```python
from build123d import *

# Parameters (mm, degrees)
SKETCH1_R           = 45
BOSS_EXTRUDE1_DEPTH = 2
SKETCH2_R           = 45
SKETCH2_R_2         = 43
BOSS_EXTRUDE2_DEPTH = 60
BOSS_EXTRUDE3_DEPTH = 20


with BuildPart() as part:
    # Sketch1 → Boss-Extrude1 (new body)
    with BuildSketch(Plane(origin=(0, 0, 0), x_dir=(1, 0, 0), z_dir=(0, 1, 0))):
        with Locations((16.5, 24.5)):
            Circle(SKETCH1_R)
    extrude(amount=BOSS_EXTRUDE1_DEPTH)

    # Sketch2 → Boss-Extrude2 (add)
    with BuildSketch(Plane(origin=(0, 2, 0), x_dir=(1, 0, 0), z_dir=(0, 1, 0))):
        with Locations((16.5, 24.5)):
            Circle(SKETCH2_R)
        with Locations((16.5, 24.5)):
            Circle(SKETCH2_R_2, mode=Mode.SUBTRACT)
    extrude(amount=BOSS_EXTRUDE2_DEPTH)

    # Sketch4 → Boss-Extrude3 (add)
    with BuildSketch(Plane(origin=(0, 2, 0), x_dir=(1, 0, 0), z_dir=(0, 1, 0))):
        with BuildLine():
            Line((16.62283723, -5.732814302), (13.748295666, -4.763073196))
            ThreePointArc((13.748295666, -4.763073196), (-7.263767503, 12.607148038), (-2.774667592, -14.282987074))
            Line((-2.774667592, -14.282987074), (13.119042931, -19.644810544))
            ThreePointArc((13.119042931, -19.644810544), (22.396673207, -14.58419971), (16.62283723, -5.732814302))
        make_face()
        with BuildLine():
            Line((13.692970384, -17.943554089), (-2.348778298, -12.531789198))
            ThreePointArc((-2.348778298, -12.531789198), (-5.619876263, 11.444627158), (11.352459564, -5.803805808))
            Line((11.352459564, -5.803805808), (16.469142545, -7.529944639))
            ThreePointArc((16.469142545, -7.529944639), (20.636876468, -14.217879696), (13.692970384, -17.943554089))
        make_face(mode=Mode.SUBTRACT)
    extrude(amount=BOSS_EXTRUDE3_DEPTH)


solid = part.part
```
The model under review builds one solid part; all positions refer to its coordinate system, in mm. A direction names the side the tool comes from. Round coordinates to 2 decimals unless told otherwise and drop trailing zeros. Order: outer loops, then holes, each group sorted by start corner. A loop starts at its lowest first (then second) coordinate and runs counter-clockwise, first axis right, second up. Notation, with made-up numbers: (84.5, -1) -> (130.5, -1) arc R19 cw to (130.5, 17) -> close; hole circle Ø5 at (-26.5, -14). An arc over 180 degrees is marked (long way). One line per item, written item: value. Start each with the question number.
Q1. Mouldability with a two-part tool opening along Z and no side actions: class faces 1 (the face through (20.667, 11.86, 14.098)), 2 (the face through (58.069, 30.566, -7.265)), 3 (the face through (16, 0, -25)) as released by +Z, released by -Z, zero draft, split by the parting line, or undercut.
Q2. Take a section at D-D (x = 3.5). Write out the cut boundary in (y, z).
Q3. Wall thickness on line 1 (X direction, y = 35.5, z = -24.5); line 2 (Z direction, x = 0, y = 8); line 3 (X direction, y = 12.5, z = 0): over which ranges is each line inside the solid? List them lowest first.
Q4. Clearance check with flat-ended pins moving along their axes: pin 1 Ø12 at (x, y) = (-13, 40) entering from -Z; pin 2 Ø1.5 at (x, z) = (-4, -20.5) entering from +Y; pin 3 Ø1.5 at (x, y) = (-5.5, 42.5) entering from -Z; pin 4 Ø10 at (x, z) = (47.5, -48.5) entering from +Y. State where each tip first meets the part, or that it passes through.
Q5. Machinability: for faces 4 (the face through (40, 62, 12)), 5 (the face through (15.206, 11.86, 5.255)), which of the approach directions +Z, -Z, +X, -X, +Y, -Y give a long, thin tool a straight path to every point of the face, cutting with its end or side? Answer none if there is none.
Q6. Take a section at B-B (x = 52). Write out the cut boundary in (y, z).
Q7. Take a section at A-A (y = 44). Write out the cut boundary in (x, z), and give its area (3 significant figures).
Q8. Take a section at C-C (z = 0). Write out the cut boundary in (x, y).
Reported:
1. face 1: undercut
1. face 2: split by the parting line
1. face 3: zero draft
2. outline: (0, -67.58) -> (62, -67.58) -> (62, -65.49) -> (2, -65.49) -> (2, -14.12) -> (22, -14.12) -> (22, -12.26) -> (2, -12.26) -> (2, 14.5) -> (22, 14.5) -> (22, 16.4) -> (2, 16.4) -> (2, 16.49) -> (62, 16.49) -> (62, 18.58) -> (0, 18.58) -> close
3. line 1: x = -28.5 to -26.5, 59.5 to 61.5
3. line 2: z = -66.37 to -64.21, -14.55 to -12.75, 13.32 to 17.37
3. line 3: x = -21.25 to -18.84, -14.55 to -12.75, 12.75 to 14.55, 51.84 to 54.25
4. pin 1: stops at z = -62.88
4. pin 2: stops at y = 2
4. pin 3: stops at z = -64.17
4. pin 4: stops at y = 62
5. face 4: +Z, -Z, +X, -X, +Y
5. face 5: +Y
6. outline: (0, -52.15) -> (62, -52.15) -> (62, -48.76) -> (2, -48.76) -> (2, -0.24) -> (62, -0.24) -> (62, 3.15) -> (0, 3.15) -> close
7. outline: circle Ø90 at (16.5, -24.5); hole circle Ø86 at (16.5, -24.5)
7. area: 553 mm2
8. outline: (-21.25, 0) -> (54.25, 0) -> (54.25, 62) -> (51.84, 62) -> (51.84, 2) -> (14.55, 2) -> (14.55, 22) -> (12.75, 22) -> (12.75, 2) -> (-12.75, 2) -> (-12.75, 22) -> (-14.55, 22) -> (-14.55, 2) -> (-18.84, 2) -> (-18.84, 62) -> (-21.25, 62) -> close
